Geometry check sheet. Reference: the model listing, model coordinates, mm. Give positions to 0.01 mm unless a question says otherwise; leave off trailing zeros. Loops run counter-clockwise (first coordinate to the right, second up) from the corner with the lowest first, then second, coordinate; pieces in that order, holes last. Notation, with made-up numbers: (-40, -22) - (-22, -22) arc R20 cw to (-22, 10) - close; hole circle Ø10 at (-15.75, 67.5). An arc over 180 degrees is marked (long way). Use a Markdown table: item, result. Add a question column.
1. Material ranges on L1, parallel to Y at x = 55, z = 1.65; L2, parallel to X at y = 64, z = 1.3; L3, parallel to Y at x = 138, z = 0.75, recorded low to high.
2. Cross-section at A-A on x = 78. Enter the section's corners in (y, z), and give its area (3 significant figures).
3. Cross-section at B-B on z = 2.05. Count the separate pieces of the cut face and the enclosed holes in it, and give its area (3 significant figures).
4. Depth check by flat-ended pin: P1, Ø0.9, axis at x = 5, z = 1.5, coming from the +Y side; P2, Ø1, axis at x = 24.5, z = 0.5, coming from the -Y side. Enter the tip coordinate at first touch or a pass-through.
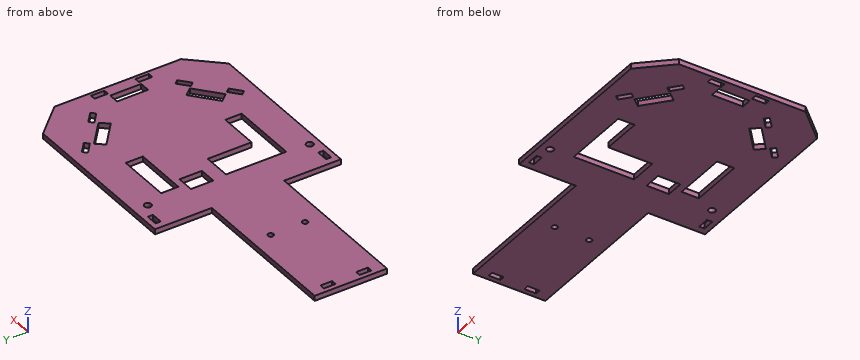
from build123d import *

# Parameters (mm, degrees)
RESSALTO_EXTRUS_O1_DEPTH = 3
ESBO_O2_W                = 31
ESBO_O2_H                = 10
ESBO_O2_W_2              = 16
ESBO_O2_H_2              = 35
ESBO_O2_W_3              = 10
ESBO_O2_H_3              = 13
ESBO_O2_W_4              = 23
ESBO_O2_H_4              = 9.5
ESBO_O2_R                = 2
CORTE_EXTRUS_O1_DEPTH    = 231.844103239
ESBO_O3_W                = 3
ESBO_O3_H                = 7.8
ESBO_O3_W_2              = 6
ESBO_O3_H_2              = 18
ESBO_O3_H_3              = 6.8
CORTE_EXTRUS_O2_DEPTH    = 10
ESBO_O4_W                = 6.8
ESBO_O4_H                = 3
CORTE_EXTRUS_O3_DEPTH    = 10
ESBO_O6_R                = 1.6
CORTE_EXTRUS_O5_DEPTH    = 10


with BuildPart() as part:
    # Esboço1 → Ressalto-extrusão1 (new body)
    with BuildSketch(Plane.XY):
        Polygon((0, 33), (0, 75), (90, 75), (90, 108), (188, 108), (204, 90.756494192), (204, 17.243505808), (188, 0), (90, 0), (90, 33), align=None)
    extrude(amount=RESSALTO_EXTRUS_O1_DEPTH)

    # Esboço2 → Corte-extrusão1 (cut, through all)
    with BuildSketch(Plane.XY.offset(3)):
        with Locations((129.5, 83.5)):
            Rectangle(ESBO_O2_W, ESBO_O2_H)
        with Locations((118, 36)):
            Rectangle(ESBO_O2_W_2, ESBO_O2_H_2)
        with Locations((114, 68)):
            Rectangle(ESBO_O2_W_3, ESBO_O2_H_3)
        with Locations((137.5, 23.25)):
            Rectangle(ESBO_O2_W_4, ESBO_O2_H_4)
        with Locations((109, 5.5)):
            Circle(ESBO_O2_R)
        with Locations((109, 99.5)):
            Circle(ESBO_O2_R)
    extrude(amount=-CORTE_EXTRUS_O1_DEPTH, mode=Mode.SUBTRACT)

    # Esboço3 → Corte-extrusão2 (cut)
    with BuildSketch(Plane.XY.offset(3)):
        Polygon((164.43729409, 6.911468095), (170.371493676, 11.973609467), (168.424516225, 14.255993924), (162.490316639, 9.193852552), align=None)
        with Locations((200.5, 41.1)):
            Rectangle(ESBO_O3_W, ESBO_O3_H)
        Polygon((190, 28.717615544), (188.053022549, 31), (182.118822963, 25.937858628), (184.065800414, 23.655474172), align=None)
        Polygon((184.065800414, 84.344525828), (190, 79.282384456), (188.053022549, 77), (182.118822963, 82.062141372), align=None)
        Polygon((162.490316639, 98.806147448), (164.43729409, 101.088531905), (170.371493676, 96.026390533), (168.424516225, 93.744006076), align=None)
        Polygon((167.126531258, 15.777583561), (180.820837996, 27.459448266), (176.926883094, 32.024217178), (163.232576357, 20.342352474), align=None)
        with Locations((200.5, 66.9)):
            Rectangle(ESBO_O3_W, ESBO_O3_H)
        with Locations((194, 54)):
            Rectangle(ESBO_O3_W_2, ESBO_O3_H_2)
        Polygon((176.926883094, 75.975782822), (163.232576357, 87.657647526), (167.126531258, 92.222416439), (180.820837996, 80.540551734), align=None)
        with Locations((4.3, 43.6)):
            Rectangle(ESBO_O3_W, ESBO_O3_H_3)
        with Locations((4.3, 64.4)):
            Rectangle(ESBO_O3_W, ESBO_O3_H_3)
    extrude(amount=-CORTE_EXTRUS_O2_DEPTH, mode=Mode.SUBTRACT)

    # Esboço4 → Corte-extrusão3 (cut)
    with BuildSketch(Plane.XY.offset(3)):
        with Locations((97.4, 103.5)):
            Rectangle(ESBO_O4_W, ESBO_O4_H)
        with Locations((97.4, 4.5)):
            Rectangle(ESBO_O4_W, ESBO_O4_H)
    extrude(amount=-CORTE_EXTRUS_O3_DEPTH, mode=Mode.SUBTRACT)

    # Esboço6 → Corte-extrusão5 (cut)
    with BuildSketch(Plane.XY.offset(3)):
        with Locations((55, 44)):
            Circle(ESBO_O6_R)
        with Locations(Location((55, 64, 0), (0, 0, 180))):
            Circle(ESBO_O6_R)
    extrude(amount=-CORTE_EXTRUS_O5_DEPTH, mode=Mode.SUBTRACT)


solid = part.part
Values found:
| question | item | result |
|---|---|---|
| 1 | L1 | y = 33 to 42.4, 45.6 to 62.4, 65.6 to 75 |
| 1 | L2 | x = 0 to 2.8, 5.8 to 53.4, 56.6 to 109, 119 to 199, 202 to 204 |
| 1 | L3 | y = 0 to 18.5, 28 to 78.5, 88.5 to 108 |
| 2 | outline | (33, 0) - (75, 0) - (75, 3) - (33, 3) - close |
| 2 | area | 126 mm2 |
| 3 | separate pieces | 1 |
| 3 | enclosed holes | 20 |
| 3 | area | 14,000 mm2 |
| 4 | P1 | stops at y = 75 |
| 4 | P2 | stops at y = 33 |
